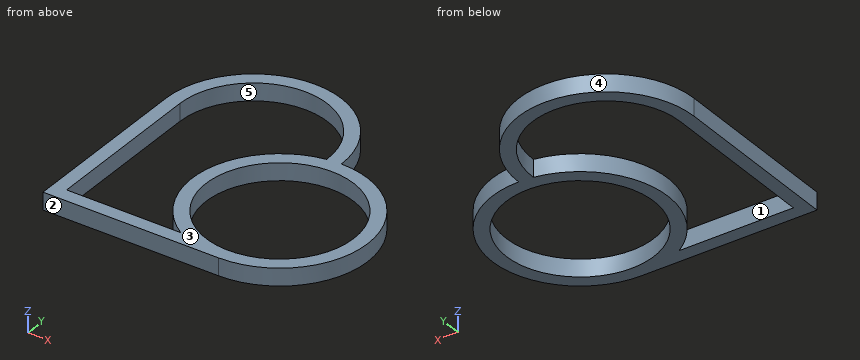
```python
from build123d import *

# Parameters (mm, degrees)
SKETCH_R  = 42.5
PAD_DEPTH = 10


with BuildPart() as part:
    # Sketch → Pad (new body)
    with BuildSketch(Plane.XY):
        with BuildLine():
            Line((-101, 0), (-101, -101))
            Line((-101, -101), (0, -101))
            ThreePointArc((0, -101), (50.5, -50.5), (0, 0))
            ThreePointArc((0, 0), (-50.5, 50.5), (-101, 0))
        make_face()
        with Locations((0, -50.5)):
            Circle(SKETCH_R, mode=Mode.SUBTRACT)
        with BuildLine():
            ThreePointArc((-8.004796, -0.638459), (-49.435348, -40.185137), (-27.276363, -93))
            Line((-93, -93), (-27.276363, -93))
            Line((-93, 0), (-93, -93))
            ThreePointArc((-8.004796, -0.638459), (-50.180761, 42.498801), (-93, 0))
        make_face(mode=Mode.SUBTRACT)
    extrude(amount=PAD_DEPTH)


solid = part.part
```
The listing builds one solid part. Answer for the finished solid, in the listing's coordinates (mm). Face numbers are marked on the shaded views. A direction names the side the tool comes from. Give positions to 0.01 mm unless a question says otherwise; leave off trailing zeros. Order: outer loops, then holes, each group sorted by start corner. A loop starts at its lowest first (then second) coordinate and runs counter-clockwise, first axis right, second up. Notation, with made-up numbers: (3.25, -28.75) -> (48.25, -28.75) arc R13 cw to (48.25, -19.75) -> close; hole circle Ø2 at (33, -32). An arc over 180 degrees is marked (long way). Answer as a JSON object with one key per item and string values. Group by question number.
Item 1: Determine the mould class of the marked faces 1, 2 and 3 for opening direction Y: pulls with the +Y half, pulls with the -Y half, needs draft (parallel to the pull), parting line crosses it, or undercut.
Item 2: The part is cut by section C-C on x = -74.5. Write down the section's boundary in (y, z).
Item 3: Consider L1, parallel to X at y = -46.5, z = 4; L2, parallel to Y at x = -13.5, z = 1.25; L3, parallel to X at y = -48, z = 5.75. Determine where each line is inside the solid, lowest interval first. Write a range as from..to.
Item 4: The part is cut by section A-A on y = -50.5. Write down the section's boundary in (x, z), and give its area (3 significant figures).
Item 5: A tool of negligible diameter and unlimited length cuts with its end or side. For the marked faces 4 and 5, from which of +Z, -Z, +X, -X, +Y, -Y can it reach the whole face along a straight path? Write none if from no direction.
Item 6: The part is cut by section D-D on x = -12.5. Write down the section's boundary in (y, z), and give its area (3 significant figures).
Item 7: Flat-ended cylindrical pins translate along their axes: pin 1 (4 mm diameter, centred on y = 18.5, z = 8.5, fed in from -X); pin 2 (4 mm diameter, centred on y = -68.5, z = 3, fed in from +X); pin 3 (1 mm diameter, centred on y = -6, z = 6, fed in from +X). Find the tip coordinate at first contact, or state that the pin passes through.
Result set:
{
 "1": {"face 1": "undercut", "face 2": "pulls with the -Y half", "face 3": "needs draft"},
 "2": {"outline": "(-101, 0) -> (-93, 0) -> (-93, 10) -> (-101, 10) -> close; (35.07, 0) -> (44.43, 0) -> (44.43, 10) -> (35.07, 10) -> close"},
 "3": {"L1": "-101..-93, -50.34..-42.31, 42.31..50.34", "L2": "-101..-90.8, -10.2..-1.84, 20.91..34.37", "L3": "-101..-93, -50.44..-42.43, 42.43..50.44"},
 "4": {"outline": "(-101, 0) -> (-93, 0) -> (-93, 10) -> (-101, 10) -> close; (-50.5, 0) -> (-42.5, 0) -> (-42.5, 10) -> (-50.5, 10) -> close; (42.5, 0) -> (50.5, 0) -> (50.5, 10) -> (42.5, 10) -> close", "area": "240 mm²"},
 "5": {"face 4": "+Z, -Z, +Y", "face 5": "+Z, -Z"},
 "6": {"outline": "(-101, 0) -> (-91.12, 0) -> (-91.12, 10) -> (-101, 10) -> close; (-9.88, 0) -> (-1.57, 0) -> (-1.57, 10) -> (-9.88, 10) -> close; (19.03, 0) -> (33.26, 0) -> (33.26, 10) -> (19.03, 10) -> close", "area": "324 mm²"},
 "7": {"pin 1": "x = -98.23", "pin 2": "x = 47.9", "pin 3": "x = 24.78"}
}
